Study the drawing (mm; zero at the part's minimum x, y, z) and answer. A direction names the side the tool comes from. Give positions to 0.01 mm unless a question says otherwise; leave off trailing zeros. Loops run counter-clockwise (first coordinate to the right, second up) from the corner with the lowest first, then second, coordinate; pieces in that order, holes last. Notation, with made-up numbers: M 87,70 L 91,70 A32 cw 91,105 Z; hole C -39,68.25 d10. An arc over 180 degrees is marked long. Use one line per item in the form item = value. Start each with the question number.
1. The part is cut by section B-B (x = 54.5). Write down the section's boundary in (y, z) (1 decimal).
2. For the marked faces 3, 4, 5 and 6, determine the directions among +Z, -Z, +X, -X, +Y, -Y from which every point of the face is accessible in a straight line to the end or side of a thin tool.
3. The mould has two halves that part along Y. Classify the marked faces 1 and 2: released by +Y, released by -Y, zero draft, split by the parting line, or undercut.
4. Straight lines are drawn through the part: line 1 (Z direction, x = 30, y = 11.75) (1 decimal); line 2 (X direction, y = 9.25, z = 43.5); line 3 (Z direction, x = 77.5, y = 12). For each, find the intervals that lie inside material, in ascending order. Write a range as from..to.
5. Each of these flat-tipped pins is pushed along its axis until it touches: pin 1 Ø2 at (y, z) = (3.5, 21) entering from -X (1 decimal); pin 2 Ø5.5 at (y, z) = (8.5, 39.5) entering from -X; pin 3 Ø5 at (x, z) = (40.5, 49.5) entering from -Y. Where does it stop, or does it pass through?
6. The part is cut by section D-D (x = 11.5). Write down the section's boundary in (y, z).
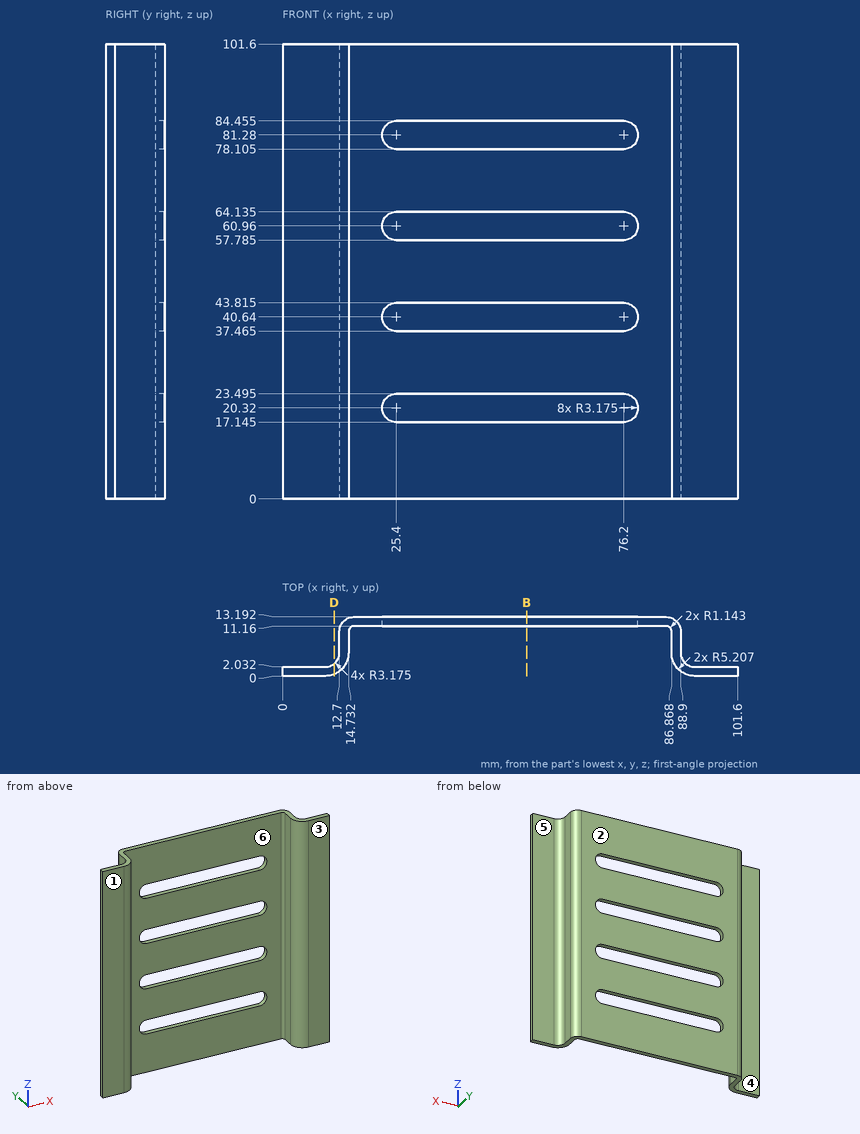
Derived:
q1.outline = M 11.2,0 L 13.2,0 L 13.2,17.1 L 11.2,17.1 Z; M 11.2,23.5 L 13.2,23.5 L 13.2,37.5 L 11.2,37.5 Z; M 11.2,43.8 L 13.2,43.8 L 13.2,57.8 L 11.2,57.8 Z; M 11.2,64.1 L 13.2,64.1 L 13.2,78.1 L 11.2,78.1 Z; M 11.2,84.5 L 13.2,84.5 L 13.2,101.6 L 11.2,101.6 Z
q2.face_3 = +Z, -Z, +X, -X, -Y
q2.face_4 = +Z, -Z, -X, +Y
q2.face_5 = +Z, -Z, +X, +Y
q2.face_6 = +Z, -Z, -Y
q3.face_1 = released by -Y
q3.face_2 = released by +Y
q4.line_1 = 0..17.1, 23.5..37.5, 43.8..57.8, 64.1..78.1, 84.5..101.6
q4.line_2 = 12.7..14.73, 86.87..88.9
q4.line_3 = 0..17.42, 23.22..37.74, 43.54..58.06, 63.86..78.38, 84.18..101.6
q5.pin_1 = 11.2
q5.pin_2 = 12.7
q5.pin_3 = 11.16
q6.outline = M 0.39,0 L 2.72,0 L 2.72,101.6 L 0.39,101.6 Z
